The listing builds one solid part. Answer for the finished solid, in the listing's coordinates (mm). Face numbers are marked on the shaded views. A direction names the side the tool comes from. Give positions to 0.01 mm unless a question says otherwise; leave off trailing zeros. Loops run counter-clockwise (first coordinate to the right, second up) from the corner with the lowest first, then second, coordinate; pieces in that order, holes last. Notation, with made-up numbers: (31.25, 0) - (66.25, 0) arc R16 cw to (66.25, 30) - close; hole circle Ø2 at (-33, -12.75). An arc over 180 degrees is marked (long way). Write item = value, one per line. Start each with the question number.
1) The part is cut by section B-B on z = 1. State how many separate pieces and enclosed holes the cut face has, plus the area to 3 significant figures.
2) Consider probe 1 along X at (y, z) = (23, 8); probe 2 along Y at (x, z) = (17, 1); probe 3 along X at (y, z) = (22, 2). Determine where each line is inside the solid, lowest interval first.
3) Flat-ended cylindrical pins translate along their axes: P1, Ø4, axis at x = -10, z = 7.5, coming from the -Y side; P2, Ø3.5, axis at y = -9, z = 2.5, coming from the -X side; P3, Ø1, axis at x = 7, z = 8, coming from the +Y side. Find the tip coordinate at first contact, or state that the pin passes through.
4) The part is cut by section D-D on x = 3. Write down the section's boundary in (y, z), plus the area to 3 significant figures.
5) Which of the six approach directions +Z, -Z, +X, -X, +Y, -Y give full straight-line access (tool end or side, diameter ignored) to the marked faces 1, 2 and 3?
6) The mould has two halves that part along Y. Classify the marked faces 4, 5 and 6: +Y half, -Y half, draft (parallel to the pull), parting line (faces both ways), or undercut.
7) The part is cut by section A-A on y = 4. Write down the section's boundary in (x, z).
8) The part is cut by section C-C on x = 16.5. Write down the section's boundary in (y, z), plus the area to 3 significant figures.
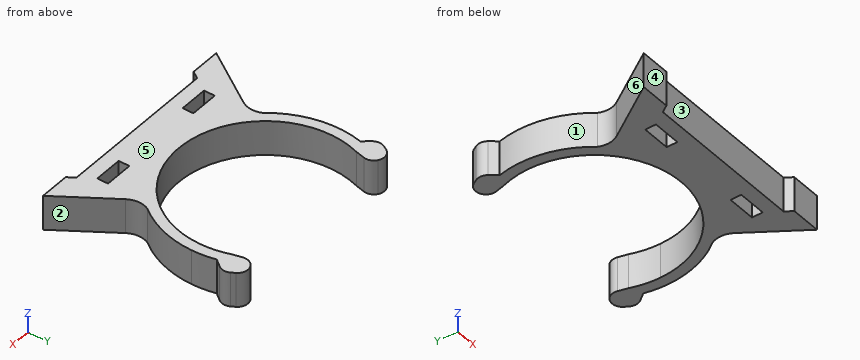
from build123d import *

# Parameters (mm, degrees)
F0_W     = 8.1
F0_H     = 3.1
F1_DEPTH = 10


with BuildPart() as f1:
    # F0 (on Top) → F1 (new body)
    with BuildSketch(Plane.XY):
        with BuildLine():
            ThreePointArc((-29.051798, 29.572342), (-29.198001, 16.866823), (-23.713784, 5.404932))
            ThreePointArc((-23.713784, 5.404932), (-1.702548, -5.093764), (20.19153, 5.647114))
            ThreePointArc((20.19153, 5.647114), (24.613354, 13.777795), (26.143006, 22.90581))
            ThreePointArc((26.143006, 22.90581), (25.940978, 26.263301), (25.33781, 29.572342))
            ThreePointArc((25.33781, 29.572342), (24.101087, 33.402381), (22.32803, 37.015544))
            ThreePointArc((22.32803, 37.015544), (21.20556, 35.608031), (21.090924, 33.811397))
            Line((21.090924, 33.811397), (21.746385, 31.144773))
            ThreePointArc((21.746385, 31.144773), (22.791378, 27.084059), (23.143006, 22.90581))
            ThreePointArc((23.143006, 22.90581), (-6.035243, -1.742562), (-25.460373, 31.144773))
            Line((-25.460373, 31.144773), (-24.804912, 33.811397))
            ThreePointArc((-24.804912, 33.811397), (-24.919548, 35.608031), (-26.042018, 37.015544))
            ThreePointArc((-26.042018, 37.015544), (-27.815075, 33.402381), (-29.051798, 29.572342))
        make_face()
        with BuildLine():
            Line((-30.676976, 31.650005), (-29.051798, 29.572342))
            ThreePointArc((-29.051798, 29.572342), (-27.815075, 33.402381), (-26.042018, 37.015544))
            ThreePointArc((-26.042018, 37.015544), (-28.392122, 37.45081), (-30.314474, 36.030595))
            Line((-30.314474, 36.030595), (-30.910288, 35.001461))
            ThreePointArc((-30.910288, 35.001461), (-31.306766, 33.290011), (-30.676976, 31.650005))
        make_face()
        with BuildLine():
            ThreePointArc((26.600486, 36.030595), (24.678134, 37.45081), (22.32803, 37.015544))
            ThreePointArc((22.32803, 37.015544), (24.101087, 33.402381), (25.33781, 29.572342))
            Line((25.33781, 29.572342), (26.962988, 31.650005))
            ThreePointArc((26.962988, 31.650005), (27.592778, 33.290011), (27.1963, 35.001461))
            Line((27.1963, 35.001461), (26.600486, 36.030595))
        make_face()
        with BuildLine():
            ThreePointArc((-23.713784, 5.404932), (-23.173383, 2.424271), (-24.15798, -0.440505))
            Line((-24.15798, -0.440505), (-34.690085, -16.299085))
            Line((-34.690085, -16.299085), (-26.101912, -16.299085))
            Line((-26.101912, -16.299085), (-24.726056, -14.227407))
            Line((-24.726056, -14.227407), (-1.856994, -14.227407))
            Line((-1.856994, -14.227407), (21.012068, -14.227407))
            Line((21.012068, -14.227407), (22.387924, -16.299085))
            Line((22.387924, -16.299085), (30.976097, -16.299085))
            Line((30.976097, -16.299085), (20.484479, -0.501468))
            ThreePointArc((20.484479, -0.501468), (19.489432, 2.532393), (20.19153, 5.647114))
            ThreePointArc((20.19153, 5.647114), (-1.702548, -5.093764), (-23.713784, 5.404932))
        make_face()
        with Locations((-18.030923, -8.677407)):
            Rectangle(F0_W, F0_H, mode=Mode.SUBTRACT)
        with Locations((14.316935, -8.677407)):
            Rectangle(F0_W, F0_H, mode=Mode.SUBTRACT)
    extrude(amount=F1_DEPTH)


solid = f1.part
Answer below:
q1.separate_pieces = 1
q1.enclosed_holes = 2
q1.area = 1,030 mm2
q2.probe_1 = -29.86 to -26.86, 23.14 to 26.14
q2.probe_2 = -14.23 to -10.23, -7.13 to 6.49
q2.probe_3 = -29.84 to -26.84, 23.13 to 26.13
q3.P1 = -14.23
q3.P2 = -31
q3.P3 = -0.28
q4.outline = (-14.23, 0) - (-1.62, 0) - (-1.62, 10) - (-14.23, 10) - close
q4.area = 126 mm2
q5.face_1 = +Z, -Z, -X
q5.face_2 = +Z, -Z, +X
q5.face_3 = +Z, -Z, -Y
q6.face_4 = -Y half
q6.face_5 = draft
q6.face_6 = undercut
q7.outline = (-23.26, 0) - (-18.21, 0) - (-18.21, 10) - (-23.26, 10) - close; (14.5, 0) - (19.6, 0) - (19.6, 10) - (14.5, 10) - close
q8.outline = (-14.23, 0) - (-10.23, 0) - (-10.23, 10) - (-14.23, 10) - close; (-7.13, 0) - (5.93, 0) - (5.93, 10) - (-7.13, 10) - close
q8.area = 171 mm2
